Source: CAD feature listing. Evaluate the final solid. Frame: model axes, mm. Coordinates: 2 decimals unless noted, no trailing zeros. Loops run counter-clockwise (first coordinate to the right, second up) from the corner with the lowest first, then second, coordinate; pieces in that order, holes last. Notation, with made-up numbers: (-22.5, 28) -> (-6.5, 28) arc R19 ccw to (-6.5, 33) -> close; hole circle Ø4 at (13, -2.5). An arc over 180 degrees is marked (long way). Answer as CSV lines item,"result".
from build123d import *

# Parameters (mm, degrees)
SKETCH1_R           = 4
BOSS_EXTRUDE1_DEPTH = 342.9
CHAMFER1_SIZE       = 0.5
SKETCH3_R           = 1.7526
CUT_EXTRUDE1_DEPTH  = 344.01663225


with BuildPart() as part:
    # Sketch1 → Boss-Extrude1 (new body)
    with BuildSketch(Plane.XY):
        Circle(SKETCH1_R)
    extrude(amount=BOSS_EXTRUDE1_DEPTH)

    # Chamfer1
    chamfer1_edges = [part.edges().sort_by_distance(p)[0] for p in [
        (-4, 0, 0),
        (-4, 0, 342.9),
    ]]
    chamfer(chamfer1_edges, length=CHAMFER1_SIZE)

    # Sketch3 → Cut-Extrude1 (cut, through all)
    with BuildSketch(Plane.ZY.offset(4)):
        with Locations((9.525, 0)):
            Circle(SKETCH3_R)
        with Locations((333.188999311, 0)):
            Circle(SKETCH3_R)
    extrude(amount=-CUT_EXTRUDE1_DEPTH, mode=Mode.SUBTRACT)


solid = part.part
(1) Cut plane B-B (z = 305.5). Return the cut outline in (x, y), then the cut area to 3 significant figures.
Computed values:
outline,"circle Ø8 at (0, 0)"
area,"50.3 mm^2"
(2) Pin query (flat end, axial travel): pin 1 Ø3 at (x, z) = (2.5, 237) entering from -Y; pin 2 Ø2 at (x, z) = (1.5, 244) entering from +Y. Return the tip coordinate at first contact, or that it passes through.
Computed values:
pin 1,"y = -3.87"
pin 2,"y = 3.97"
(3) Cut plane A-A (y = 0). Return the cut outline in (x, z), then the cut area to 3 significant figures.
Computed values:
outline,"(-4, 0.5) -> (-3.5, 0) -> (3.5, 0) -> (4, 0.5) -> (4, 7.77) -> (-4, 7.77) -> close; (-4, 11.28) -> (4, 11.28) -> (4, 331.44) -> (-4, 331.44) -> close; (-4, 334.94) -> (4, 334.94) -> (4, 342.4) -> (3.5, 342.9) -> (-3.5, 342.9) -> (-4, 342.4) -> close"
area,"2,690 mm^2"
(4) Material intervals for L1, parallel to Z at x = 0.5, y = 0; L2, parallel to Z at x = 2, y = -0.75; L3, parallel to Y at x = -0.5, z = 49, sorted ascending. Write a range as [from, to].
Computed values:
L1,"[0, 7.77], [11.28, 331.44], [334.94, 342.9]"
L2,"[0, 7.94], [11.11, 331.6], [334.77, 342.9]"
L3,"[-3.97, 3.97]"
